from build123d import *

# Parameters (mm, degrees)
SKETCH20_R          = 2.350664171
BOSS_EXTRUDE1_DEPTH = 0.5
CHAMFER1_SIZE       = 0.2


with BuildPart() as part:
    # Sketch19 → Revolve1 (revolve)
    with BuildSketch(Plane.XY, mode=Mode.PRIVATE) as revolve1_sk:
        with BuildLine():
            Line((1.80625, 1.491762035), (2.813920411, 1.125))
            Line((2.813920411, 1.125), (10.99725, 1.125))
            Line((10.99725, 1.125), (10.99725, 1.28276631))
            ThreePointArc((10.99725, 1.28276631), (10.941275199, 1.440418529), (10.798416223, 1.527474335))
            Line((10.798416223, 1.527474335), (6.866483245, 2.349605776))
            ThreePointArc((6.866483245, 2.349605776), (6.824719556, 2.339469211), (6.80625, 2.300664171))
            Line((6.80625, 2.300664171), (6.80625, 2))
            ThreePointArc((6.80625, 2), (6.733026695, 1.823223305), (6.55625, 1.75))
            Line((6.55625, 1.75), (2.55625, 1.75))
            ThreePointArc((2.55625, 1.75), (2.379473305, 1.823223305), (2.30625, 2))
            Line((2.30625, 2), (2.30625, 2.75))
            Line((2.30625, 2.75), (1.80625, 2.75))
            Line((1.80625, 2.75), (1.80625, 1.491762035))
        make_face()
    revolve(revolve1_sk.sketch.rotate(Axis((0, 0, 0), (1, 0, 0)), 90), axis=Axis((0, 0, 0), (1, 0, 0)))  # turned: the seam where the file's is

    # Sketch20 → Boss-Extrude1 (add)
    with BuildSketch(Plane(origin=(2.30625, 0, 0), x_dir=(0, 0, -1), z_dir=(1, 0, 0))):
        with BuildLine():
            Line((-3.7747, 2.775), (3.7747, 2.775))
            ThreePointArc((3.7747, 2.775), (4.826521337, 2.339321337), (5.2622, 1.2875))
            Line((5.2622, 1.2875), (5.2622, -3.7747))
            ThreePointArc((5.2622, -3.7747), (4.826521337, -4.826521337), (3.7747, -5.2622))
            Line((3.7747, -5.2622), (-3.7747, -5.2622))
            ThreePointArc((-3.7747, -5.2622), (-4.826521337, -4.826521337), (-5.2622, -3.7747))
            Line((-5.2622, -3.7747), (-5.2622, 1.2875))
            ThreePointArc((-5.2622, 1.2875), (-4.826521337, 2.339321337), (-3.7747, 2.775))
        make_face()
        Circle(SKETCH20_R, mode=Mode.SUBTRACT)
    extrude(amount=-BOSS_EXTRUDE1_DEPTH)

    # Chamfer1
    chamfer1_edges = [part.edges().sort_by_distance(p)[0] for p in [
        (1.80625, 2.339321337, -4.826521337),
        (1.80625, -1.2436, -5.2622),
        (1.80625, -4.826521337, -4.826521337),
        (1.80625, -5.2622, 0),
        (1.80625, -4.826521337, 4.826521337),
        (1.80625, -1.2436, 5.2622),
        (1.80625, 2.339321337, 4.826521337),
        (1.80625, 2.775, 0),
    ]]
    chamfer(chamfer1_edges, length=CHAMFER1_SIZE)


solid = part.part
The listing builds one solid part. Answer for the finished solid, in the listing's coordinates (mm). Coordinates: 2 decimals unless noted, no trailing zeros. Loops run counter-clockwise (first coordinate to the right, second up) from the corner with the lowest first, then second, coordinate; pieces in that order, holes last.
1) Find the intervals of material crossed by L1, parallel to Y at x = 5.5, z = 0 (3 decimals); L2, parallel to X at y = -0.25, z = -3.75; L3, parallel to Y at x = 8, z = 0 (3 decimals), in increasing order.
2) Flat-ended cylindrical pins translate along their axes: pin 1 Ø3 at (y, z) = (0, 0) entering from +X; pin 2 Ø4 at (x, y) = (10, 1.5) entering from +Z; pin 3 Ø5 at (x, z) = (8.5, 3.5) entering from +Y; pin 4 Ø5 at (x, z) = (5.5, 0) entering from +Y. Find the tip coordinate at first contact, or state that the pin passes through.
3) Find section A-A on z = 0. Write down the section's boundary in (x, y) (3 decimals).
4) Find section C-C on y = -2.5. Write down the section's boundary in (x, z).
5) Determine the mould class of faces 1 (the face through (6.96, -0.76, -0.83)), 2 (the face through (9.242, -1.837, -0.241)), 3 (the face through (1.806, -2, 0)) for opening direction Y: pulls with the +Y half, pulls with the -Y half, needs draft (parallel to the pull), parting line crosses it, or undercut.
6) Find section D-D on z = 3. Write down the section's boundary in (x, y) (3 decimals), then the cut area to 3 significant figures.
7) Find section B-B on y = 0. Write down the section's boundary in (x, z) (3 decimals).
Values:
1. L1: y = -1.75 to -1.125, 1.125 to 1.75
1. L2: x = 1.81 to 2.31
1. L3: y = -2.113 to -1.125, 1.125 to 2.113
2. pin 1: stops at x = 11
2. pin 2: stops at z = 2.01
2. pin 3: stops at y = 1.86
2. pin 4: stops at y = 2.35
3. outline: (1.806, -5.062) - (2.006, -5.262) - (2.306, -5.262) - (2.306, -2) arc R0.25 cw to (2.556, -1.75) - (6.556, -1.75) arc R0.25 cw to (6.806, -2) - (6.806, -2.301) arc R0.05 ccw to (6.866, -2.35) - (10.798, -1.527) arc R0.25 ccw to (10.997, -1.283) - (10.997, -1.125) - (2.814, -1.125) - (1.806, -1.492) - close; (1.806, 1.492) - (2.814, 1.125) - (10.997, 1.125) - (10.997, 1.283) arc R0.25 ccw to (10.798, 1.527) - (6.866, 2.35) arc R0.05 ccw to (6.806, 2.301) - (6.806, 2) arc R0.25 cw to (6.556, 1.75) - (2.556, 1.75) arc R0.25 cw to (2.306, 2) - (2.306, 2.775) - (2.006, 2.775) - (1.806, 2.575) - close
4. outline: (1.81, -5.06) - (2.01, -5.26) - (2.31, -5.26) - (2.31, 5.26) - (2.01, 5.26) - (1.81, 5.06) - close
5. face 1: undercut
5. face 2: parting line crosses it
5. face 3: needs draft
6. outline: (1.806, -5.062) - (2.006, -5.262) - (2.306, -5.262) - (2.306, 2.775) - (2.006, 2.775) - (1.806, 2.575) - close
6. area: 3.98 mm2
7. outline: (1.806, -5.062) - (2.006, -5.262) - (2.306, -5.262) - (2.306, -2) arc R0.25 cw to (2.556, -1.75) - (6.556, -1.75) arc R0.25 cw to (6.806, -2) - (6.806, -2.301) arc R0.05 ccw to (6.866, -2.35) - (10.798, -1.527) arc R0.25 ccw to (10.997, -1.283) - (10.997, -1.125) - (2.814, -1.125) - (1.806, -1.492) - close; (1.806, 1.492) - (2.814, 1.125) - (10.997, 1.125) - (10.997, 1.283) arc R0.25 ccw to (10.798, 1.527) - (6.866, 2.35) arc R0.05 ccw to (6.806, 2.301) - (6.806, 2) arc R0.25 cw to (6.556, 1.75) - (2.556, 1.75) arc R0.25 cw to (2.306, 2) - (2.306, 5.262) - (2.006, 5.262) - (1.806, 5.062) - close
